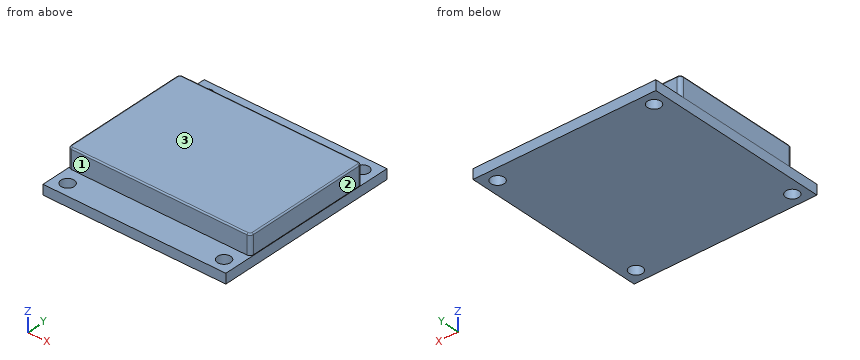
```python
from build123d import *

# Parameters (mm, degrees)
F0_W     = 27.7
F0_H     = 28.2
F0_R     = 1
F2_DEPTH = 1.5
F3_W     = 27.6
F3_H     = 19.46
F4_DEPTH = 3
F5_R     = 0.5
F6_R     = 0.2


with BuildPart() as f2:
    # F0 (on Top) → F2 (new body)
    with BuildSketch(Plane.XY):
        with Locations((0.0295223769, -0.0248048455)):
            Rectangle(F0_W, F0_H)
        with Locations((-11.8204776231, -12.1248048455)):
            Circle(F0_R, mode=Mode.SUBTRACT)
        with Locations((11.8795223769, -12.1248048455)):
            Circle(F0_R, mode=Mode.SUBTRACT)
        with Locations((-11.8204776231, 12.0751951545)):
            Circle(F0_R, mode=Mode.SUBTRACT)
        with Locations((11.8795223769, 12.0751951545)):
            Circle(F0_R, mode=Mode.SUBTRACT)
    extrude(amount=F2_DEPTH)

    # F3 (on face) → F4 (join)
    with BuildSketch(Plane.XY.offset(1.5)):
        Rectangle(F3_W, F3_H)
    extrude(amount=F4_DEPTH)

    # F5
    f5_edges = [f2.edges().sort_by_distance(p)[0] for p in [
        (13.8, -9.73, 3),
        (13.8, 9.73, 3),
        (-13.8, 9.73, 3),
        (-13.8, -9.73, 3),
    ]]
    fillet(f5_edges, radius=F5_R)

    # F6
    f6_edges = [f2.edges().sort_by_distance(p)[0] for p in [
        (0, 9.73, 4.5),
        (13.653553, 9.583553, 4.5),
        (-13.653553, 9.583553, 4.5),
        (13.8, 0, 4.5),
        (-13.8, 0, 4.5),
        (13.653553, -9.583553, 4.5),
        (-13.653553, -9.583553, 4.5),
        (0, -9.73, 4.5),
    ]]
    fillet(f6_edges, radius=F6_R)


solid = f2.part
```
Input: part model. Units: mm. Frame: model coordinates. Face numbers are marked on the shaded views. A direction names the side the tool comes from. Give positions to 0.01 mm unless a question says otherwise; leave off trailing zeros. Order: outer loops, then holes, each group sorted by start corner. A loop starts at its lowest first (then second) coordinate and runs counter-clockwise, first axis right, second up. Notation, with made-up numbers: (64, 73) -> (77, 73) arc R7 cw to (77, 81) -> close; hole circle Ø6 at (-38.75, -8). An arc over 180 degrees is marked (long way). Write each question's results on one line, items separated by ' | '. Start each with the question number.
Item 1: Cut plane D-D on z = 0.8. Return the cut outline in (x, y).
Item 2: Cut plane A-A on z = 2.85. Return the cut outline in (x, y), then the cut area to 3 significant figures.
Item 3: Contact query for flat-ended pins moving along their axis: P1, Ø1.4, axis at y = 4.5, z = 2.5, coming from the -X side; P2, Ø1.2, axis at x = 11.88, y = 12.08, coming from the +Z side; P3, Ø2.5, axis at x = -11.82, y = 12.08, coming from the +Z side; P4, Ø1.5, axis at x = 7.5, z = 3, coming from the +Y side. Output: stop coordinate, or through.
Item 4: Cut plane C-C on x = -1.75. Return the cut outline in (y, z), then the cut area to 3 significant figures.
Item 5: Line query: line 1 (Y direction, x = 1.75, z = 3.3); line 2 (Z direction, x = 11.5, y = 11); line 3 (X direction, y = -0.5, z = 2.9). Output: solid intervals per line, ascending.
Item 6: Set-up query: the marked faces 1, 2 and 3. Return all of +Z, -Z, +X, -X, +Y, -Y with unobstructed straight access to the full face (end or side cutting, diameter ignored); none if empty.
Item 7: Cut plane B-B on y = 12.5. Return the cut outline in (x, z), then the cut area to 3 significant figures.
Established:
1) outline: (-13.82, -14.12) -> (13.88, -14.12) -> (13.88, 14.08) -> (-13.82, 14.08) -> close; hole circle Ø2 at (-11.82, -12.12); hole circle Ø2 at (-11.82, 12.08); hole circle Ø2 at (11.88, -12.12); hole circle Ø2 at (11.88, 12.08)
2) outline: (-13.8, -9.23) arc R0.5 ccw to (-13.3, -9.73) -> (13.3, -9.73) arc R0.5 ccw to (13.8, -9.23) -> (13.8, 9.23) arc R0.5 ccw to (13.3, 9.73) -> (-13.3, 9.73) arc R0.5 ccw to (-13.8, 9.23) -> close | area: 537 mm^2
3) P1: x = -13.8 | P2: through | P3: z = 1.5 | P4: y = 9.73
4) outline: (-14.12, 0) -> (14.08, 0) -> (14.08, 1.5) -> (9.73, 1.5) -> (9.73, 4.3) arc R0.2 ccw to (9.53, 4.5) -> (-9.53, 4.5) arc R0.2 ccw to (-9.73, 4.3) -> (-9.73, 1.5) -> (-14.12, 1.5) -> close | area: 101 mm^2
5) line 1: -9.73 to 9.73 | line 2: 0 to 1.5 | line 3: -13.8 to 13.8
6) face 1: +Z, +X, -X, -Y | face 2: +Z, +X, +Y, -Y | face 3: +Z, +X, -X, +Y, -Y
7) outline: (-13.82, 0) -> (-12.73, 0) -> (-12.73, 1.5) -> (-13.82, 1.5) -> close; (-10.92, 0) -> (10.97, 0) -> (10.97, 1.5) -> (-10.92, 1.5) -> close; (12.78, 0) -> (13.88, 0) -> (13.88, 1.5) -> (12.78, 1.5) -> close | area: 36.1 mm^2
